Read the model definition and answer for the solid it produces. Units are mm, in the model's axes. Face numbers are marked on the shaded views. A direction names the side the tool comes from. Coordinates: 2 decimals unless noted, no trailing zeros. Loops run counter-clockwise (first coordinate to the right, second up) from the corner with the lowest first, then second, coordinate; pieces in that order, holes last. Notation, with made-up numbers: (52.5, 6) - (101.5, 6) arc R20 ccw to (101.5, 30) - close; hole circle Ø10 at (-11.5, 46). An arc over 180 degrees is marked (long way). Use one line per item in the form item = value.
from build123d import *

# Parameters (mm, degrees)
F0_R     = 1.8
F1_DEPTH = 17
F2_DEPTH = 20
F5_DEPTH = 6.6367971034


with BuildPart() as f1:
    # F0 (on Top) → F1 (new body)
    with BuildSketch(Plane.XY):
        with BuildLine():
            ThreePointArc((-9, -11.048189897), (-6.1160649114, 12.8707517263), (14.25, 0))
            ThreePointArc((14.25, 0), (12.8707517263, -6.1160649114), (9, -11.048189897))
            Line((9, -11.048189897), (9, -18.7594200464))
            ThreePointArc((9, -18.7594200464), (17.6093087314, -11.0827833364), (20.8066297242, 0))
            ThreePointArc((20.8066297242, 0), (-11.0827833364, 17.6093087314), (-9, -18.7594200464))
            Line((-9, -18.7594200464), (-9, -11.048189897))
        make_face()
        with Locations((-17.45, 0)):
            Circle(F0_R, mode=Mode.SUBTRACT)
        with Locations((17.45, 0)):
            Circle(F0_R, mode=Mode.SUBTRACT)
        with Locations((17.45, 0)):
            Circle(F0_R)
        with Locations((-17.45, 0)):
            Circle(F0_R)
    extrude(amount=F1_DEPTH)

    # F0 (on Top) → F2 (join)
    with BuildSketch(Plane.XY):
        with Locations((17.45, 0)):
            Circle(F0_R)
        with Locations((-17.45, 0)):
            Circle(F0_R)
    extrude(amount=F2_DEPTH)

    # F4 (on plane+point) → F5 (cut, through all)
    with BuildSketch(Plane.YZ.offset(-20.8066297242)):
        with BuildLine():
            Line((1.5, 7.5), (1.5, 11.5))
            ThreePointArc((1.5, 11.5), (0, 12), (-1.5, 11.5))
            Line((-1.5, 11.5), (-1.5, 7.5))
            ThreePointArc((-1.5, 7.5), (0, 7), (1.5, 7.5))
        make_face()
    extrude(amount=F5_DEPTH, mode=Mode.SUBTRACT)


solid = f1.part
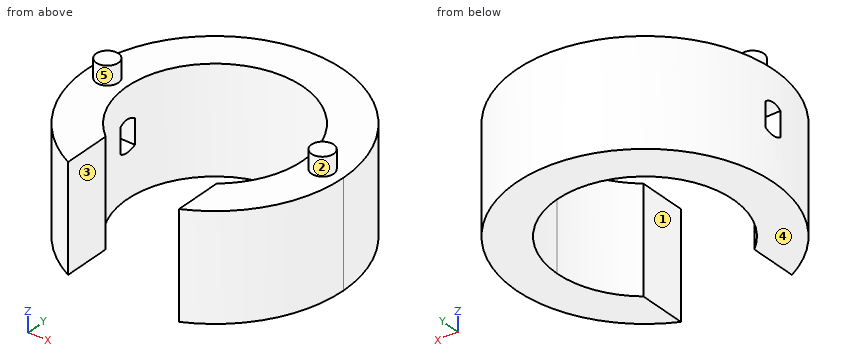
Item 1: Find the intervals of material crossed by L1, parallel to Y at x = 0, z = 9.5; L2, parallel to X at y = -0.5, z = 16.5; L3, parallel to X at y = -4, z = 8.75, in increasing order.
Results below:
L1 = 14.25 to 20.81
L2 = -20.8 to -14.24, 14.24 to 20.8
L3 = -20.42 to -13.68, 13.68 to 20.42
Item 2: The part is cut by section C-C on y = -5. Give the vertices of the cut face in (x, z), plus the area to 3 significant figures.
Results below:
outline = (-20.2, 0) - (-13.34, 0) - (-13.34, 17) - (-20.2, 17) - close; (13.34, 0) - (20.2, 0) - (20.2, 17) - (13.34, 17) - close
area = 233 mm²
Item 3: For a pull along X with two mould halves and no side action, classify the marked faces 3, 4 and 5 as +X half, -X half, draft (parallel to the pull), parting line (faces both ways), or undercut.
Results below:
face_3 = undercut
face_4 = draft
face_5 = undercut
Item 4: The part is cut by section B-B on z = 17.75. Give the vertices of the cut face in (x, y), plus the area to 3 significant figures.
Results below:
outline = circle Ø3.6 at (-17.45, 0); circle Ø3.6 at (17.45, 0)
area = 20.4 mm²
Item 5: Each of these flat-tipped pins is pushed along its axis until it touches: P1, Ø8.5, axis at y = -14, z = 8.5, coming from the +X side; P2, Ø20, axis at x = -1.5, y = -1, coming from the +Z side; P3, Ø6, axis at y = 13.5, z = 3.5, coming from the +X side; P4, Ø2, axis at x = -17.5, z = 8.5, coming from the -Y side. Where does it stop, or does it pass through?
Results below:
P1 = 18.38
P2 = through
P3 = 17.96
P4 = -12.68
Item 6: The part is cut by section A-A on x = -11.5. Give the vertices of the cut face in (y, z), plus the area to 3 significant figures.
Results below:
outline = (-17.34, 0) - (-8.42, 0) - (-8.42, 17) - (-17.34, 17) - close; (8.42, 0) - (17.34, 0) - (17.34, 17) - (8.42, 17) - close
area = 303 mm²
Item 7: Which of the six approach directions +Z, -Z, +X, -X, +Y, -Y give full straight-line access (tool end or side, diameter ignored) to the marked faces 1 and 2?
Results below:
face_1 = +Z, -Z, -Y
face_2 = +Z
Item 8: The part is cut by section D-D on x = 0. Give the vertices of the cut face in (y, z), plus the area to 3 significant figures.
Results below:
outline = (14.25, 0) - (20.81, 0) - (20.81, 17) - (14.25, 17) - close
area = 111 mm²
